Autodesk Fusion 360 part; units mm, degrees
sketch "Sketch1" plane through (0, 0, 0) normal (0, 1, 0) x (1, 0, 0)
  line L0 (0, -300) -> (259.8076, -150)
  line L1 (259.8076, -150) -> (259.8076, 150)
  line L2 (259.8076, 150) -> (0, 300)
  line L3 (0, 300) -> (-259.8076, 150)
  line L4 (-259.8076, 150) -> (-259.8076, -150)
  line L5 (-259.8076, -150) -> (0, -300)
  dimension "d1" = 300
extrude "Extrude1" add sketch "Sketch1" along normal blind 5
sketch "Sketch2" plane through (0, 5, 0) normal (0, 1, 0) x (-1, 0, 0)
  line L0 (259.8076, 150) -> (0, 300)
  line L1 (0, 300) -> (-259.8076, 150)
  line L2 (-259.8076, 150) -> (-259.8076, -150)
  line L3 (-259.8076, -150) -> (0, -300)
  line L4 (0, -300) -> (259.8076, -150)
  line L5 (259.8076, -150) -> (259.8076, 150)
Model file for the job. Use its own axes, mm. Give positions to 0.01 mm unless a question says otherwise; leave off trailing zeros. Order: outer loops, then holes, each group sorted by start corner. A loop starts at its lowest first (then second) coordinate and runs counter-clockwise, first axis right, second up. Notation, with made-up numbers: (-18.75, 63.5) -> (39.25, 63.5) arc R15 ccw to (39.25, 75.5) -> close; hole circle Ø11 at (59.5, 50.5). An arc over 180 degrees is marked (long way). Use CSV: the item, a comma, the result in double quotes.
1. Band-saw the part on A-A, the plane y = 2.8. Give the cut face in (x, z).
Outcome:
outline,"(-259.81, -150) -> (0, -300) -> (259.81, -150) -> (259.81, 150) -> (0, 300) -> (-259.81, 150) -> close"
2. Drop flat-ended pins along their axis: pin 1 (6 mm diameter, centred on x = 195.5, z = 12, fed in from -Y); pin 2 (1.5 mm diameter, centred on y = 3, z = -183.5, fed in from +X). Give the stop position or say it passes through.
Outcome:
pin 1,"y = 0"
pin 2,"x = 203.08"
3. Band-saw the part on C-C, the plane z = -207.5. Give the cut face in (x, y), then the cut area to 3 significant figures.
Outcome:
outline,"(-160.21, 0) -> (160.21, 0) -> (160.21, 5) -> (-160.21, 5) -> close"
area,"1,600 mm²"
4. Mould opens along Y. For faces 1 (the flat face through (-131.72, 2.46, 223.95)), 2 (the flat face through (-4, 5, -4)), 3 (the flat face through (-4, 0, -4)) say: +Y half, -Y half, draft (parallel to the pull), parting line (faces both ways), or undercut.
Outcome:
face 1,"draft"
face 2,"+Y half"
face 3,"-Y half"
5. Drill centre lines: line 1 along X through (y, z) = (3, 197.5); line 2 along X through (y, z) = (2.5, 198.5); line 3 along Z through (x, y) = (38, 4). Where is each one in solid material? Low to high. Write a range as from..to.
Outcome:
line 1,"-177.54..177.54"
line 2,"-175.8..175.8"
line 3,"-278.06..278.06"
6. Band-saw the part on B-B, the plane x = 85. Give the cut face in (y, z), then the cut area to 3 significant figures.
Outcome:
outline,"(0, -250.93) -> (5, -250.93) -> (5, 250.93) -> (0, 250.93) -> close"
area,"2,510 mm²"
